For this review, take the finished solid that the model builds, in its own axes (mm). Face numbers are marked on the shaded views. A direction names the side the tool comes from. Coordinates: 2 decimals unless noted, no trailing zeros. Loops run counter-clockwise (first coordinate to the right, second up) from the corner with the lowest first, then second, coordinate; pieces in that order, holes last. Notation, with made-up numbers: (-8.75, -17) -> (3.25, -17) arc R21 ccw to (3.25, 6) -> close; hole circle Ø10 at (68.5, 47.25). An arc over 180 degrees is marked (long way). One line per item, written item: value.
from build123d import *

# Parameters (mm, degrees)
SKETCH1_R           = 3.81
BOSS_EXTRUDE1_DEPTH = 2.54
SKETCH2_R           = 1.905
CUT_EXTRUDE2_DEPTH  = 1.27
SKETCH3_W           = 5.369563314
SKETCH3_H           = 5.391171223
BOSS_EXTRUDE2_DEPTH = 12.7
SKETCH4_W           = 3.561314924
SKETCH4_H           = 2.408690502
CUT_EXTRUDE3_DEPTH  = 12.7


with BuildPart() as part:
    # Sketch1 → Boss-Extrude1 (new body)
    with BuildSketch(Plane(origin=(0, 0, 0), x_dir=(1, 0, 0), z_dir=(0, 1, 0))):
        with Locations(Location((0, 0, 0), (0, 0, 270))):
            Circle(SKETCH1_R)
    extrude(amount=BOSS_EXTRUDE1_DEPTH)

    # Sketch2 → Cut-Extrude2 (cut)
    with BuildSketch(Plane.XZ):
        with Locations(Location((0, 0, 0), (0, 0, 270))):
            Circle(SKETCH2_R)
    extrude(amount=-CUT_EXTRUDE2_DEPTH, mode=Mode.SUBTRACT)

    # Sketch3 → Boss-Extrude2 (add)
    with BuildSketch(Plane(origin=(0, 2.54, 0), x_dir=(1, 0, 0), z_dir=(0, 1, 0))):
        with Locations((0.012751297, 0.004969332)):
            Rectangle(SKETCH3_W, SKETCH3_H)
    extrude(amount=BOSS_EXTRUDE2_DEPTH)

    # Sketch4 → Cut-Extrude3 (cut)
    with BuildSketch(Plane(origin=(2.697532954, 0, 0), x_dir=(0, 0, -1), z_dir=(1, 0, 0))):
        with Locations((0.026120509, 13.211421801)):
            Rectangle(SKETCH4_W, SKETCH4_H)
    extrude(amount=-CUT_EXTRUDE3_DEPTH, mode=Mode.SUBTRACT)


solid = part.part
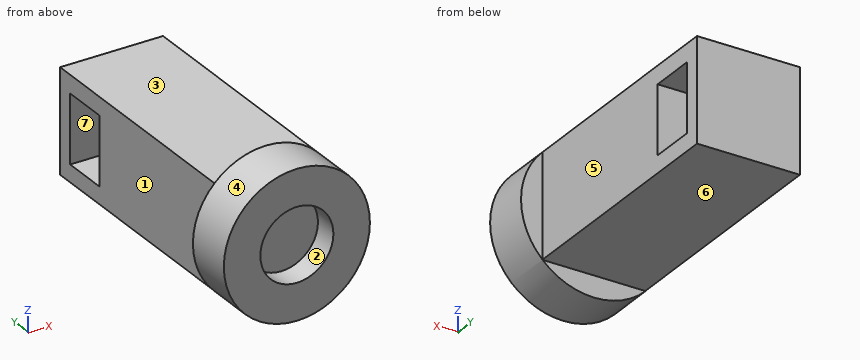
1. Take a section at B-B, the plane y = 12.5. Give the boundary of the cut face in (x, z), and give its area (3 significant figures).
Return value:
outline: (-2.67, -2.7) -> (2.7, -2.7) -> (2.7, -1.81) -> (-2.67, -1.81) -> close; (-2.67, 1.75) -> (2.7, 1.75) -> (2.7, 2.69) -> (-2.67, 2.69) -> close
area: 9.83 mm2
2. The part is to be moulded in two halves that separate along X. For the marked faces 1, 2, 3 and 4, say which applies: pulls with the +X half, pulls with the -X half, needs draft (parallel to the pull), parting line crosses it, or undercut.
Return value:
face 1: pulls with the -X half
face 2: undercut
face 3: needs draft
face 4: parting line crosses it
3. Take a section at A-A, the plane x = 0. Give the boundary of the cut face in (y, z) (3 decimals).
Return value:
outline: (0, -3.81) -> (2.54, -3.81) -> (2.54, -2.701) -> (15.24, -2.701) -> (15.24, 2.691) -> (2.54, 2.691) -> (2.54, 3.81) -> (0, 3.81) -> (0, 1.905) -> (1.27, 1.905) -> (1.27, -1.905) -> (0, -1.905) -> close; hole (12.007, -1.807) -> (14.416, -1.807) -> (14.416, 1.755) -> (12.007, 1.755) -> close
4. To check wall thickness, follow probe 1 along X at (y, z) = (0.6, 0) (3 decimals); probe 2 along Y at (x, z) = (-0.25, -1); probe 3 along Y at (x, z) = (-2.5, -1.5). State the ranges of each line that lie inside material, in increasing order. Write a range as from..to.
Return value:
probe 1: x = -3.81..-1.905, 1.905..3.81
probe 2: y = 1.27..12.01, 14.42..15.24
probe 3: y = 0..12.01, 14.42..15.24
5. Insertion check: pin 1 Ø3 at (x, z) = (2, 1.5) entering from -Y; pin 2 Ø1.5 at (y, z) = (2, 1.5) entering from +X; pin 3 Ø1.2 at (x, y) = (-1.5, 14) entering from +Z; pin 4 Ø3 at (y, z) = (5, 2) entering from +X. Each pin has a flat end and moves straight along its axis. Give the tip position at first contact, or say it passes through.
Return value:
pin 1: stops at y = 0
pin 2: stops at x = 3.74
pin 3: stops at z = 2.69
pin 4: stops at x = 2.7
6. Take a section at C-C, the plane z = 0. Give the boundary of the cut face in (x, y) (3 decimals), and give its area (3 significant figures).
Return value:
outline: (-3.81, 0) -> (-1.905, 0) -> (-1.905, 1.27) -> (1.905, 1.27) -> (1.905, 0) -> (3.81, 0) -> (3.81, 2.54) -> (2.698, 2.54) -> (2.698, 12.007) -> (-2.672, 12.007) -> (-2.672, 2.54) -> (-3.81, 2.54) -> close; (-2.672, 14.416) -> (2.698, 14.416) -> (2.698, 15.24) -> (-2.672, 15.24) -> close
area: 69.8 mm2
7. Take a section at D-D, the plane x = -1.25. Give the boundary of the cut face in (y, z), and give its area (3 significant figures).
Return value:
outline: (0, -3.6) -> (2.54, -3.6) -> (2.54, -2.7) -> (15.24, -2.7) -> (15.24, 2.69) -> (2.54, 2.69) -> (2.54, 3.6) -> (0, 3.6) -> (0, 1.44) -> (1.27, 1.44) -> (1.27, -1.44) -> (0, -1.44) -> close; hole (12.01, -1.81) -> (14.42, -1.81) -> (14.42, 1.75) -> (12.01, 1.75) -> close
area: 74.5 mm2
8. For the marked faces 5, 6 and 7, list the 3-axis set-ups (+Z, -Z, +X, -X, +Y, -Y) from which the entire face can be reached by the end or side of a thin tool; tool diameter is ignored.
Return value:
face 5: +Z, -Z, +X, +Y
face 6: -Z, +X, -X, +Y
face 7: +X, -X
